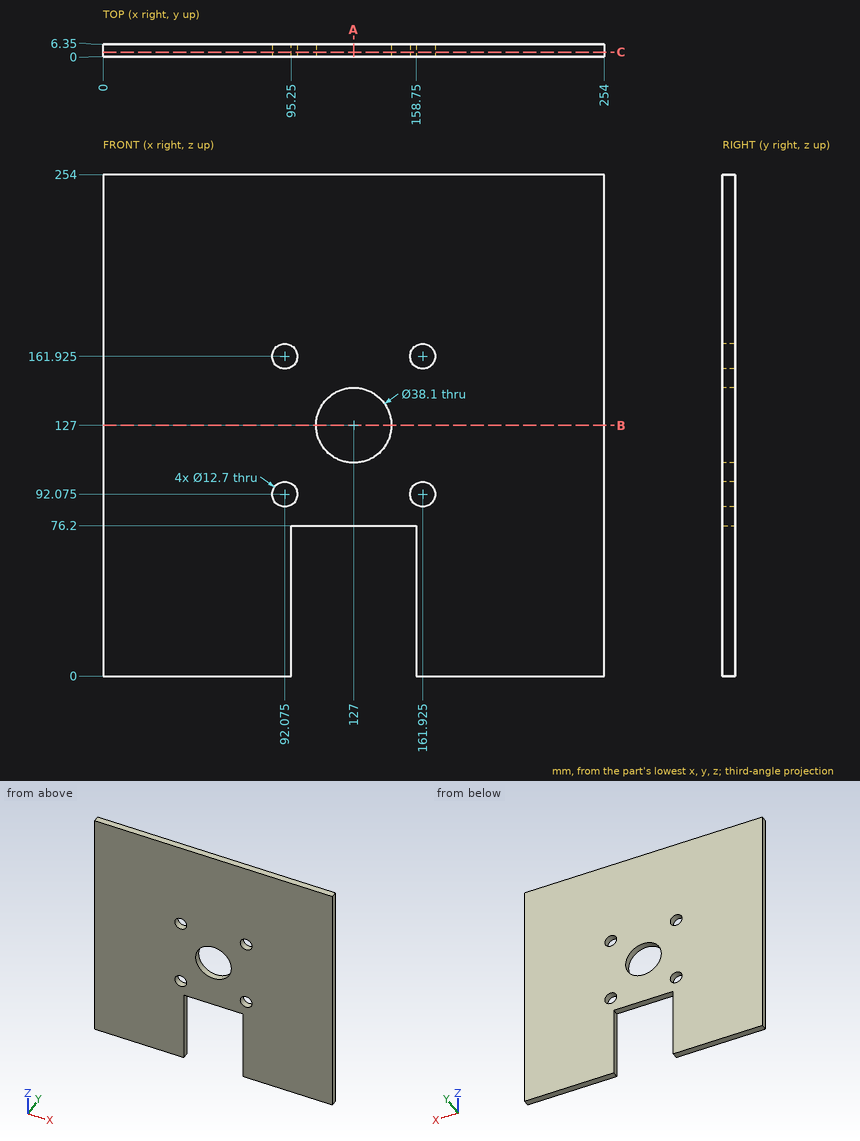
Can you work these out from the drawing? Everything is in mm from the part's minimum corner. Give positions to 0.01 mm unless a question says otherwise; leave off trailing zeros. Order: outer loops, then holes, each group sorted by start corner. A loop starts at its lowest first (then second) coordinate and runs counter-clockwise, first axis right, second up. Notation, with made-up numbers: M 3,6 L 43,6 A25 ccw 43,28 Z; hole C -29,-4 d1. An arc over 180 degrees is marked long. Use a Markdown table: item, result. Add a question column.
Item 1: If I drill on L1, parallel to X at y = 4, z = 31; L2, parallel to X at y = 4, z = 94; L3, parallel to X at y = 3.25, z = 127, over which ranges is the centre line in solid material (lowest first)? Write a range as [from, to].
Item 2: Suppose I cut it at C-C (y = 2.25). List the corners of the cut face in (x, z) for me (3 decimals).
Item 3: Suppose I cut it at A-A (x = 127). List the corners of the cut face in (y, z) for me.
Item 4: Will these pins go through, and if not, where does the flat tip stop? pin 1 (7.5 mm diameter, centred on x = 92.075, z = 92.075, fed in from -Y); pin 2 (1.5 mm diameter, centred on x = 114.5, y = 1, fed in from -Z).
Item 5: Suppose I cut it at B-B (z = 127). List the corners of the cut face in (x, y) for me.
Answer sheet:
| question | item | result |
|---|---|---|
| 1 | L1 | x = [0, 95.25], [158.75, 254] |
| 1 | L2 | x = [0, 86.02], [98.13, 155.87], [167.98, 254] |
| 1 | L3 | x = [0, 107.95], [146.05, 254] |
| 2 | outline | M 0,0 L 95.25,0 L 95.25,76.2 L 158.75,76.2 L 158.75,0 L 254,0 L 254,254 L 0,254 Z; hole C 92.075,92.075 d12.7; hole C 92.075,161.925 d12.7; hole C 127,127 d38.1; hole C 161.925,92.075 d12.7; hole C 161.925,161.925 d12.7 |
| 3 | outline | M 0,76.2 L 6.35,76.2 L 6.35,107.95 L 0,107.95 Z; M 0,146.05 L 6.35,146.05 L 6.35,254 L 0,254 Z |
| 4 | pin 1 | passes through |
| 4 | pin 2 | stops at z = 76.2 |
| 5 | outline | M 0,0 L 107.95,0 L 107.95,6.35 L 0,6.35 Z; M 146.05,0 L 254,0 L 254,6.35 L 146.05,6.35 Z |
